Job drawing, mm, ordinate dimensions from the low corner. One solid piece. A direction names the side the tool comes from. Give positions to 0.01 mm unless a question says otherwise; leave off trailing zeros. Loops run counter-clockwise (first coordinate to the right, second up) from the corner with the lowest first, then second, coordinate; pieces in that order, holes last. Notation, with made-up numbers: M 61,27.5 L 67,27.5 A20 ccw 67,34.5 Z; hole C 62.25,-17.5 d10. An arc over 180 degrees is marked long. Answer as CSV lines item,"result".
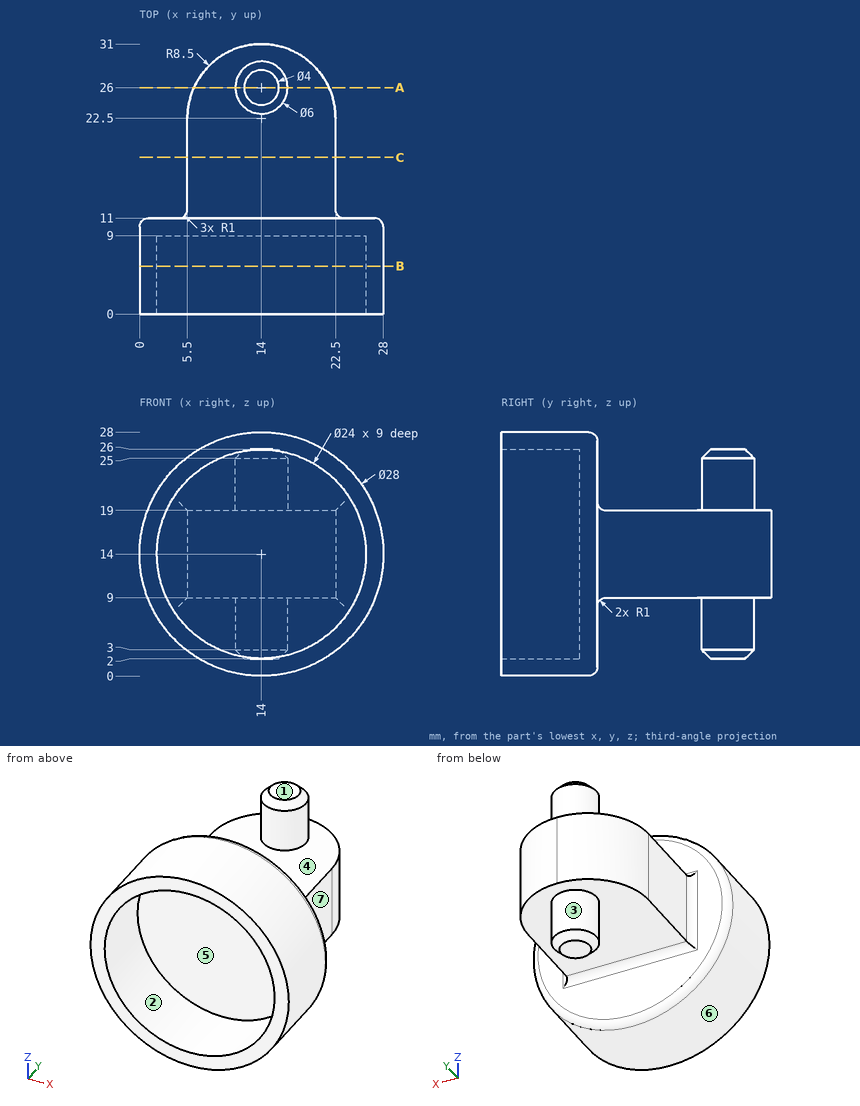
1) Drill centre lines: line 1 (X direction, y = 2, z = 14); line 2 (Z direction, x = 20, y = 26); line 3 (Y direction, x = 21.75, z = 14.5). Where is each one in solid material? Low to high. Write a range as from..to.
Answer below:
line 1,"x = 0..2, 26..28"
line 2,"z = 9..19"
line 3,"y = 9..25.99"
2) Band-saw the part on B-B on y = 5.5. Give the cut face in (x, z), and give its area (3 significant figures).
Answer below:
outline,"C 14,14 d28; hole C 14,14 d24"
area,"163 mm^2"
3) Band-saw the part on A-A on y = 26. Give the cut face in (x, z), and give its area (3 significant figures).
Answer below:
outline,"M 6.25,9 L 11,9 L 11,3 L 12,2 L 16,2 L 17,3 L 17,9 L 21.75,9 L 21.75,19 L 17,19 L 17,25 L 16,26 L 12,26 L 11,25 L 11,19 L 6.25,19 Z"
area,"237 mm^2"
4) Flat gauge pins, fed straight in: pin 1 (5 mm diameter, centred on x = 17, y = 20, fed in from +Z); pin 2 (11 mm diameter, centred on y = 18.5, z = 14.5, fed in from -X); pin 3 (10 mm diameter, centred on x = 19.5, z = 6.5, fed in from +Y). Where does each tip first touch, or does it go through?
Answer below:
pin 1,"stops at z = 19"
pin 2,"stops at x = 5.5"
pin 3,"stops at y = 30.92"
5) Which spindle directions (+Z, -Z, +X, -X, +Y, -Y) get a long thin tool onto all of the face, cutting with end or side? Do the marked faces 1, 2, 3 and 4. Say none if no direction does.
Answer below:
face 1,"+Z, +X, -X, +Y"
face 2,"-Y"
face 3,"-Z"
face 4,"+Z"
6) Band-saw the part on C-C on y = 18. Give the cut face in (x, z).
Answer below:
outline,"M 5.5,9 L 22.5,9 L 22.5,19 L 5.5,19 Z"
7) Mould opens along Z. For the marked faces 5, 6 and 7 say: +Z half, -Z half, draft (parallel to the pull), parting line (faces both ways), or undercut.
Answer below:
face 5,"undercut"
face 6,"parting line"
face 7,"draft"
